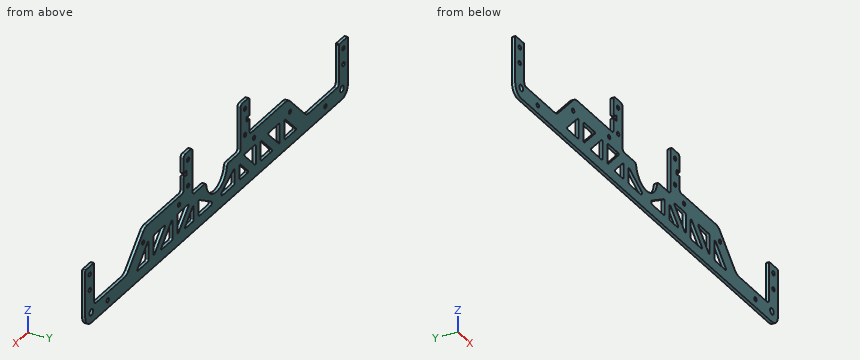
from build123d import *

# Parameters (mm, degrees)
EXTRUDE_1_DEPTH     = 3
SKETCH_2_R          = 2
SKETCH_2_W          = 80
SKETCH_2_H          = 45
SKETCH_2_W_2        = 5
SKETCH_2_H_2        = 3
CUT_EXTRUDE_1_DEPTH = 10
SKETCH_5_R          = 3
SKETCH_5_R_2        = 17.5
SKETCH_5_R_3        = 1
CUT_EXTRUDE_4_DEPTH = 234.518735865
CUT_EXTRUDE_5_DEPTH = 234.518735865
FILLET_1_R          = 10
FILLET_2_R          = 3
FILLET_3_R          = 1
FILLET_4_R          = 2


with BuildPart() as part:
    # 草图1 → 凸台-拉伸1 (new body)
    with BuildSketch(Plane(origin=(0, 0, 0), x_dir=(1, 0, 0), z_dir=(0, 1, 0))):
        with BuildLine():
            Line((-55, 0), (55, 0))
            Line((55, 0), (55, 35.5))
            Line((55, 35.5), (119.5, 35.5))
            Line((119.5, 35.5), (150, 66))
            Line((150, 66), (204, 66))
            Line((204, 66), (204, 26))
            Line((204, 26), (219, 26))
            Line((219, 26), (219, 71))
            ThreePointArc((219, 71), (216.071067812, 78.071067812), (209, 81))
            Line((209, 81), (-209, 81))
            ThreePointArc((-209, 81), (-216.071067812, 78.071067812), (-219, 71))
            Line((-219, 71), (-219, 26))
            Line((-219, 26), (-204, 26))
            Line((-204, 26), (-204, 66))
            Line((-204, 66), (-150, 66))
            Line((-150, 66), (-119.5, 35.5))
            Line((-119.5, 35.5), (-55, 35.5))
            Line((-55, 35.5), (-55, 0))
        make_face()
    extrude(amount=EXTRUDE_1_DEPTH)

    # 草图2 → 切除-拉伸1 (cut)
    with BuildSketch(Plane(origin=(0, 3, 0), x_dir=(1, 0, 0), z_dir=(0, 1, 0))):
        with Locations(Location((-47.5, 32.5, 0), (0, 0, 270))):
            Circle(SKETCH_2_R)
        with Locations(Location((-211.5, 33.5, 0), (0, 0, 270))):
            Circle(SKETCH_2_R)
        with Locations(Location((-211.5, 48.5, 0), (0, 0, 270))):
            Circle(SKETCH_2_R)
        with Locations(Location((211.5, 48.5, 0), (0, 0, 270))):
            Circle(SKETCH_2_R)
        with Locations(Location((211.5, 33.5, 0), (0, 0, 270))):
            Circle(SKETCH_2_R)
        with Locations(Location((-181.5, 73.5, 0), (0, 0, 270))):
            Circle(SKETCH_2_R)
        with Locations(Location((181.5, 73.5, 0), (0, 0, 270))):
            Circle(SKETCH_2_R)
        with Locations(Location((47.5, 32.5, 0), (0, 0, 270))):
            Circle(SKETCH_2_R)
        with Locations(Location((-47.5, 7.5, 0), (0, 0, 270))):
            Circle(SKETCH_2_R)
        with Locations(Location((-62.5, 43, 0), (0, 0, 270))):
            Circle(SKETCH_2_R)
        with Locations(Location((-122.5, 48.5, 0), (0, 0, 270))):
            Circle(SKETCH_2_R)
        with Locations(Location((62.5, 43, 0), (0, 0, 270))):
            Circle(SKETCH_2_R)
        with Locations(Location((122.5, 48.5, 0), (0, 0, 270))):
            Circle(SKETCH_2_R)
        with Locations(Location((47.5, 7.5, 0), (0, 0, 270))):
            Circle(SKETCH_2_R)
        with Locations((0, 22.5)):
            Rectangle(SKETCH_2_W, SKETCH_2_H)
        with Locations((52.5, 19)):
            Rectangle(SKETCH_2_W_2, SKETCH_2_H_2)
        with Locations((-52.5, 19)):
            Rectangle(SKETCH_2_W_2, SKETCH_2_H_2)
    extrude(amount=-CUT_EXTRUDE_1_DEPTH, mode=Mode.SUBTRACT)

    # 草图5 → 切除-拉伸4 (cut, through all)
    with BuildSketch(Plane(origin=(0, 3, 0), x_dir=(1, 0, 0), z_dir=(0, 1, 0))):
        with Locations(Location((-209, 71, 0), (0, 0, 270))):
            Circle(SKETCH_5_R)
        with Locations(Location((209, 71, 0), (0, 0, 90))):
            Circle(SKETCH_5_R)
        with Locations((0, 45)):
            Circle(SKETCH_5_R_2)
        with Locations((-51, 20.5)):
            Circle(SKETCH_5_R_3)
        with Locations((-51, 17.5)):
            Circle(SKETCH_5_R_3)
        with Locations((51, 17.5)):
            Circle(SKETCH_5_R_3)
        with Locations((51, 20.5)):
            Circle(SKETCH_5_R_3)
    extrude(amount=-CUT_EXTRUDE_4_DEPTH, mode=Mode.SUBTRACT)

    # 草图6 → 切除-拉伸5 (cut, through all)
    with BuildSketch(Plane(origin=(0, 3, 0), x_dir=(1, 0, 0), z_dir=(0, 1, 0))):
        Polygon((-133.786796564, 71), (-113.286796564, 71), (-113.286796564, 50.5), align=None)
        Polygon((-105.286796564, 50.5), (-105.286796564, 71), (-84.786796564, 50.5), align=None)
        with BuildLine():
            Line((-30.159379566, 71), (-9.91066826, 71))
            ThreePointArc((-9.91066826, 71), (-7.978816608, 69.51763809), (-8.91066826, 67.267949192))
            Line((-8.91066826, 67.267949192), (-30.159379566, 55))
            Line((-30.159379566, 55), (-30.159379566, 71))
        make_face()
        Polygon((84.786796564, 50.5), (105.286796564, 50.5), (105.286796564, 71), align=None)
        Polygon((113.286796564, 50.5), (133.786796564, 71), (113.286796564, 71), align=None)
        Polygon((-93.973088065, 71), (-73.473088065, 71), (-73.473088065, 50.5), align=None)
        Polygon((-65.473088065, 50.5), (-65.473088065, 71), (-44.973088065, 50.5), align=None)
        Polygon((-54.159379566, 71), (-38.159379566, 71), (-38.159379566, 55), align=None)
        Polygon((38.159379566, 55), (54.159379566, 71), (38.159379566, 71), align=None)
        Polygon((44.973088065, 50.5), (65.473088065, 50.5), (65.473088065, 71), align=None)
        Polygon((73.473088065, 50.5), (93.973088065, 71), (73.473088065, 71), align=None)
        with BuildLine():
            Line((30.159379566, 55), (30.159379566, 71))
            Line((30.159379566, 71), (9.91066826, 71))
            ThreePointArc((9.91066826, 71), (7.978816608, 69.51763809), (8.91066826, 67.267949192))
            Line((8.91066826, 67.267949192), (30.159379566, 55))
        make_face()
    extrude(amount=-CUT_EXTRUDE_5_DEPTH, mode=Mode.SUBTRACT)

    # 圆角1
    fillet_1_edges = [part.edges().sort_by_distance(p)[0] for p in [
        (-119.5, 1.5, -35.5),
        (-150, 1.5, -66),
        (150, 1.5, -66),
        (119.5, 1.5, -35.5),
    ]]
    fillet(fillet_1_edges, radius=FILLET_1_R)

    # 圆角2
    fillet_2_edges = [part.edges().sort_by_distance(p)[0] for p in [
        (17.5, 1.5, -45),
        (-17.5, 1.5, -45),
        (55, 1.5, 0),
        (-55, 1.5, 0),
        (-55, 1.5, -35.5),
        (-204, 1.5, -66),
        (204, 1.5, -66),
        (55, 1.5, -35.5),
        (-40, 1.5, 0),
        (-40, 1.5, -45),
        (40, 1.5, -45),
        (40, 1.5, 0),
    ]]
    fillet(fillet_2_edges, radius=FILLET_2_R)

    # 圆角3
    fillet_3_edges = [part.edges().sort_by_distance(p)[0] for p in [
        (55, 1.5, -17.5),
        (55, 1.5, -20.5),
        (-55, 1.5, -17.5),
        (-55, 1.5, -20.5),
        (-113.286796564, 1.5, -50.5),
        (-133.786796564, 1.5, -71),
        (113.286796564, 1.5, -50.5),
        (133.786796564, 1.5, -71),
        (84.786796564, 1.5, -50.5),
        (105.286796564, 1.5, -71),
        (30.159379566, 1.5, -55),
        (-38.159379566, 1.5, -55),
        (-54.159379566, 1.5, -71),
        (-204, 1.5, -26),
        (-219, 1.5, -26),
        (-73.473088065, 1.5, -50.5),
        (-93.973088065, 1.5, -71),
        (219, 1.5, -26),
        (204, 1.5, -26),
        (-30.159379566, 1.5, -55),
        (-84.786796564, 1.5, -50.5),
        (-105.286796564, 1.5, -71),
        (73.473088065, 1.5, -50.5),
        (93.973088065, 1.5, -71),
        (44.973088065, 1.5, -50.5),
        (65.473088065, 1.5, -71),
        (38.159379566, 1.5, -55),
        (54.159379566, 1.5, -71),
        (-44.973088065, 1.5, -50.5),
        (-65.473088065, 1.5, -71),
    ]]
    fillet(fillet_3_edges, radius=FILLET_3_R)

    # 圆角4
    fillet_4_edges = [part.edges().sort_by_distance(p)[0] for p in [
        (-113.286796564, 1.5, -71),
        (113.286796564, 1.5, -71),
        (105.286796564, 1.5, -50.5),
        (30.159379566, 1.5, -71),
        (-38.159379566, 1.5, -71),
        (-73.473088065, 1.5, -71),
        (-30.159379566, 1.5, -71),
        (-105.286796564, 1.5, -50.5),
        (73.473088065, 1.5, -71),
        (65.473088065, 1.5, -50.5),
        (38.159379566, 1.5, -71),
        (-65.473088065, 1.5, -50.5),
    ]]
    fillet(fillet_4_edges, radius=FILLET_4_R)


solid = part.part
For this review, take the finished solid that the model builds, in its own axes (mm). Give positions to 0.01 mm unless a question says otherwise; leave off trailing zeros. Write each loop counter-clockwise with the first axis right and the second up, starting at its lowest first coordinate (ties: lowest second). Pieces come first, ordered by that corner, then holes. Notation, with made-up numbers: (84.25, 54) -> (106.25, 54) arc R21 ccw to (106.25, 69) -> close; hole circle Ø11 at (5.5, -35.75). An arc over 180 degrees is marked (long way). Use CSV: the item, a comma, the result in double quotes.
Q1. Take a section at A-A, the plane y = 1.4. State how many separate pieces and enclosed holes the cut face has, then the cut area to 3 significant figures.
Conclusion:
separate pieces,"1"
enclosed holes,"28"
area,"13,200 mm2"
Q2. Take a section at B-B, the plane x = 167. Write out the cut boundary in (y, z), then the cut area to 3 significant figures.
Conclusion:
outline,"(0, -81) -> (3, -81) -> (3, -66) -> (0, -66) -> close"
area,"45.0 mm2"
Q3. For P1, Ø0.9, axis at x = -89.5, y = 1, coming from the +Z side; P2, Ø1.5, axis at x = -27, y = 2, coming from the +Z side, all flat-tipped, find the tip position at first contact; note any pin that passes through.
Conclusion:
P1,"z = -35.5"
P2,"z = -45"
Q4. To check wall thickness, follow probe 1 along Z at (x, y) = (-181.5, 0.9); probe 2 along Z at (x, y) = (-53.5, 0.4); probe 3 along Z at (x, y) = (211.5, 2.2). State the ranges of each line that lie inside material, in increasing order. Write a range as [from, to].
Conclusion:
probe 1,"[-81, -75.5], [-71.5, -66]"
probe 2,"[-81, -59.03], [-50.5, -20.5], [-17.5, -0.4]"
probe 3,"[-80.68, -72.66], [-69.34, -50.5], [-46.5, -35.5], [-31.5, -26]"
